Autodesk Inventor part; units mm, degrees
ref_plane "YZ Plane" through (0, 0, 0) normal (1, 0, 0) x (0, 1, 0)
ref_plane "XZ Plane" through (0, 0, 0) normal (0, 1, 0) x (-1, 0, 0)
ref_plane "XY Plane" through (0, 0, 0) normal (0, 0, 1) x (1, 0, 0)
sketch "Sketch1" plane through (0, 0, 0) normal (0, 0, 1) x (1, 0, 0)
  circle A0 centre (0, 0) radius 4.25
  dimension "d0" = 8.5
extrude "Extrusion1" add sketch "Sketch1" along normal blind 5
sketch "Sketch2" plane through (0, 0, 5) normal (0, 0, 1) x (1, 0, 0)
  circle A0 centre (0, 0) radius 4.25
  circle A1 centre (0, 0) radius 2.5
  dimension "d3" = 5
extrude "Extrusion2" add sketch "Sketch2" along normal blind 30 contours A1
sketch "Sketch3" plane through (0, 0, 0) normal (0, 0, -1) x (-1, 0, 0)
  circle A0 centre (0, 0) radius 4.25
  line L0 (2.3094, 0) -> (1.1547, -2)
  line L1 (1.1547, -2) -> (-1.1547, -2)
  line L2 (-1.1547, -2) -> (-2.3094, 0)
  line L3 (-2.3094, 0) -> (-1.1547, 2)
  line L4 (-1.1547, 2) -> (1.1547, 2)
  line L5 (1.1547, 2) -> (2.3094, 0)
  dimension "d6" = 4
extrude "Extrusion3" cut sketch "Sketch3" against normal blind 3 contours L0 L1 L2 L3 L4 L5
thread "Thread1"
properties part number "m5x0.8"
Verification items for the finished model (mm, model axes). A direction names the side the tool comes from. Coordinates: 2 decimals unless noted, no trailing zeros. Order: outer loops, then holes, each group sorted by start corner. A loop starts at its lowest first (then second) coordinate and runs counter-clockwise, first axis right, second up. Notation, with made-up numbers: (76, 9.25) -> (83, 9.25) arc R31 ccw to (83, 42.25) -> close; hole circle Ø4 at (-0.75, -16.75). An arc over 180 degrees is marked (long way). Answer as CSV lines item,"result". Start each with the question number.
1) Cross-section at D-D, the plane x = -3. Record the boundary of the cut face in (y, z).
2) Set-up check for faces 4 (the face through (1.724, -1.014, 1.479)), 5 (the face through (2, -1, 0)), 6 (the face through (2, -2, 5)): record each of +Z, -Z, +X, -X, +Y, -Y from which the full face is reachable in a straight line by a thin tool's end or side.
3) Cross-section at A-A, the plane x = 0. Record the boundary of the cut face in (y, z).
4) Cross-section at C-C, the plane z = 15. Record the boundary of the cut face in (x, y).
5) Release check for a two-part mould opening along X. For faces 1 (the face through (-0.54, 2.44, 19.79)), 2 (the face through (0, 0, 3)), 3 (the face through (0, 0, 35)) record: released by +X, released by -X, zero draft, split by the parting line, or undercut.
6) Gauge pin test, flat ends, axial feed: pin 1 Ø1.5 at (x, z) = (0, 25) entering from -Y; pin 2 Ø2 at (x, y) = (0.5, 0) entering from -Z; pin 3 Ø4 at (x, z) = (3, 7.5) entering from -Y. Record the tip position at first contact, or that the pin passes through.
7) Cross-section at B-B, the plane y = -0.75. Record the boundary of the cut face in (x, z), then the cut area to 3 significant figures.
8) Material ranges on L1, parallel to Z at x = 1.75, y = 0.5; L2, parallel to Z at x = -2.25, y = -2.75; L3, parallel to Y at x = 1.5, z = 14, recorded low to high. Write a range as [from, to].
Conclusion:
1,outline,"(-3.01, 0) -> (3.01, 0) -> (3.01, 5) -> (-3.01, 5) -> close"
2,face 4,"-Z"
2,face 5,"-Z, +X, -X, +Y, -Y"
2,face 6,"+Z"
3,outline,"(-4.25, 0) -> (-2, 0) -> (-2, 3) -> (2, 3) -> (2, 0) -> (4.25, 0) -> (4.25, 5) -> (2.5, 5) -> (2.5, 35) -> (-2.5, 35) -> (-2.5, 5) -> (-4.25, 5) -> close"
4,outline,"circle Ø5 at (0, 0)"
5,face 1,"split by the parting line"
5,face 2,"undercut"
5,face 3,"zero draft"
6,pin 1,"stops at y = -2.5"
6,pin 2,"stops at z = 3"
6,pin 3,"stops at y = -2.29"
7,outline,"(-4.18, 0) -> (-1.88, 0) -> (-1.88, 3) -> (1.88, 3) -> (1.88, 0) -> (4.18, 0) -> (4.18, 5) -> (2.38, 5) -> (2.38, 35) -> (-2.38, 35) -> (-2.38, 5) -> (-4.18, 5) -> close"
7,area,"174 mm²"
8,L1,"z = [3, 35]"
8,L2,"z = [0, 5]"
8,L3,"y = [-2, 2]"
